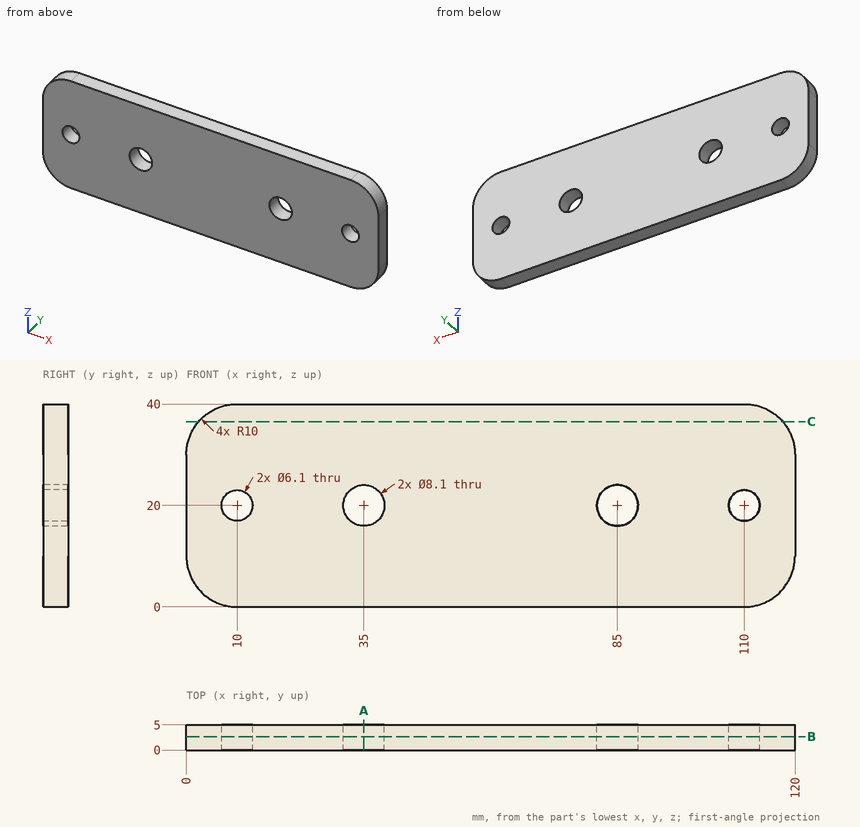
Geometry: see drawing. Coordinates: mm, zero at the bounding-box minimum. Give positions to 0.01 mm unless a question says otherwise; leave off trailing zeros. Order: outer loops, then holes, each group sorted by start corner. A loop starts at its lowest first (then second) coordinate and runs counter-clockwise, first axis right, second up. Notation, with made-up numbers: M -13,21 L 7,21 A21 cw 7,50 Z; hole C -39,6 d2. An arc over 180 degrees is marked long. Answer as CSV lines item,"result". Start each with the question number.
1) First-contact query: P1, Ø1, axis at x = 20, y = 2.5, coming from the -Z side. Flat tip, straight axial feed; report the tip coordinate or a pass-through.
2) Line query: line 1 (X direction, y = 3.65, z = 20); line 2 (Z direction, x = 85, y = 1.3); line 3 (X direction, y = 2.35, z = 18). Output: solid intervals per line, ascending. Write a range as from..to.
3) Cut plane B-B (y = 2.7). Output: boundary loops of the cut face in (x, z).
4) Cut plane C-C (z = 36.5). Output: boundary loops of the cut face in (x, y), then the cut area to 3 significant figures.
5) Cut plane A-A (x = 35). Output: boundary loops of the cut face in (y, z), then the cut area to 4 significant figures.
Findings below:
1,P1,"stops at z = 0"
2,line 1,"x = 0..6.95, 13.05..30.95, 39.05..80.95, 89.05..106.95, 113.05..120"
2,line 2,"z = 0..15.95, 24.05..40"
2,line 3,"x = 0..7.7, 12.3..31.48, 38.52..81.48, 88.52..107.7, 112.3..120"
3,outline,"M 0,10 A10 ccw 10,0 L 110,0 A10 ccw 120,10 L 120,30 A10 ccw 110,40 L 10,40 A10 ccw 0,30 Z; hole C 10,20 d6.1; hole C 35,20 d8.1; hole C 85,20 d8.1; hole C 110,20 d6.1"
4,outline,"M 2.4,0 L 117.6,0 L 117.6,5 L 2.4,5 Z"
4,area,"576 mm²"
5,outline,"M 0,0 L 5,0 L 5,15.95 L 0,15.95 Z; M 0,24.05 L 5,24.05 L 5,40 L 0,40 Z"
5,area,"159.5 mm²"
